Autodesk Inventor part; units mm, degrees
ref_plane "YZ Plane" through (0, 0, 0) normal (1, 0, 0) x (0, 1, 0)
ref_plane "XZ Plane" through (0, 0, 0) normal (0, 1, 0) x (-1, 0, 0)
ref_plane "XY Plane" through (0, 0, 0) normal (0, 0, 1) x (1, 0, 0)
sketch "Sketch1" plane through (0, 0, 0) normal (0, 0, 1) x (1, 0, 0)
  line L0 (0, 0) -> (0, -152.4)
  line L1 (76.2, -152.4) -> (76.2, 0)
  arc A0 (0, -152.4) -> (76.2, -152.4) centre (38.1, -152.4) ccw
  arc A1 (76.2, 0) -> (0, 0) centre (38.1, 0) ccw
  circle A2 centre (38.1, 0) radius 1.5875
  circle A3 centre (38.1, -152.4) radius 1.5875
  dimension "d17" = 3.175
  dimension "d18" = 3.175
extrude "Extrusion1" add sketch "Sketch1" along normal blind 6.35 contours A1 L1 A0 L0 | A2 | A3
extrude "Extrusion4" cut sketch "Sketch1" along normal blind 12.7 contours A2 | A3
sketch "Sketch3" plane through (0, 0, 6.35) normal (0, 0, 1) x (1, 0, 0)
  arc A0 (0, -152.4) -> (76.2, -152.4) centre (38.1, -152.4) ccw
  line L0 (38.1, -190.5) -> (38.1, -187.325)
  arc A1 (3.175, -152.4) -> (38.1, -187.325) centre (38.1, -152.4) ccw
  arc A2 (76.2, 0) -> (0, 0) centre (38.1, 0) ccw
  line L1 (38.1, 38.1) -> (38.1, 34.925)
  arc A3 (38.1, 34.925) -> (3.175, 0) centre (38.1, 0) ccw
  line L2 (3.175, -152.4) -> (3.175, 0)
  line L3 (0, 0) -> (0, -152.4)
  dimension "d21" = 3.175
  dimension "d23" = 3.175
  dimension "d24" = 3.175
extrude "Extrusion5" add sketch "Sketch3" along normal blind 12.7
sketch "Sketch4" plane through (0, 0, 6.35) normal (0, 0, 1) x (1, 0, 0)
  point P0 (0, 0)
properties part number "ChainGuard"
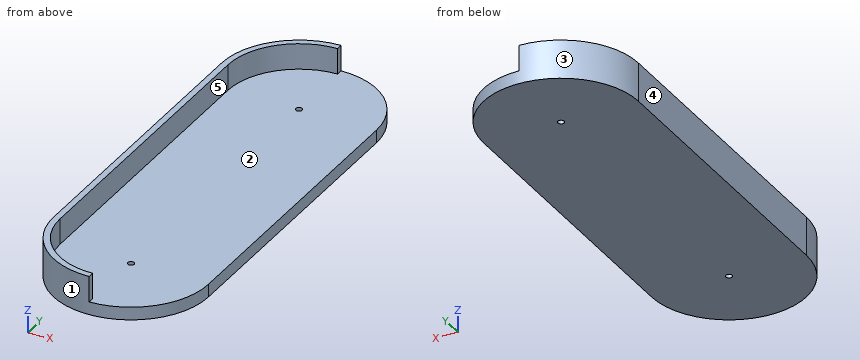
Part model, mm, in its own coordinate system. Face numbers are marked on the shaded views. A direction names the side the tool comes from. Coordinates: 2 decimals unless noted, no trailing zeros. Order: outer loops, then holes, each group sorted by start corner. A loop starts at its lowest first (then second) coordinate and runs counter-clockwise, first axis right, second up.
(1) Slice it at B-B, the plane y = -115. Write the cut outline in (x, z) (3 decimals).
Check sheet entries:
outline: (0, 0) - (76.2, 0) - (76.2, 6.35) - (3.175, 6.35) - (3.175, 19.05) - (0, 19.05) - close
(2) Pull direction Y, two halves, no side cores. Call the marked faces 1, 2 and 3: pulls with the +Y half, pulls with the -Y half, needs draft (parallel to the pull), parting line crosses it, or undercut.
Check sheet entries:
face 1: pulls with the -Y half
face 2: undercut
face 3: pulls with the +Y half
(3) Tool access for the marked faces 4 and 5: list every direction of +Z, -Z, +X, -X, +Y, -Y with a clear straight run to the whole face (end or side of a thin tool).
Check sheet entries:
face 4: +Z, -Z, -X, +Y, -Y
face 5: +Z, +X
(4) Probe L1, parallel to Y at x = 38.1, z = 1.5; L2, parallel to X at y = 0, z = 3.5; L3, parallel to Z at x = 10, y = 13. List the from-to ranges inside material, lowest first.
Check sheet entries:
L1: y = -190.5 to -153.99, -150.81 to -1.59, 1.59 to 38.1
L2: x = 0 to 36.51, 39.69 to 76.2
L3: z = 0 to 6.35
(5) Slice it at A-A, the plane z = 16.5. Write the cut outline in (x, y) (3 decimals).
Check sheet entries:
outline: (0, -152.4) arc R38.1 ccw to (38.1, -190.5) - (38.1, -187.325) arc R34.925 cw to (3.175, -152.4) - (3.175, 0) arc R34.925 cw to (38.1, 34.925) - (38.1, 38.1) arc R38.1 ccw to (0, 0) - close
(6) Pin check, flat tips, straight feed: pin 1 Ø2.5 at (x, y) = (38.1, 0) entering from -Z; pin 2 Ø10 at (x, z) = (63, 5) entering from +Y; pin 3 Ø22 at (x, y) = (39, -117) entering from +Z; pin 4 Ø10 at (x, z) = (13.5, 13.5) entering from +Y. Stop position of each tip, or through.
Check sheet entries:
pin 1: passes through
pin 2: stops at y = 32.49
pin 3: stops at z = 6.35
pin 4: stops at y = 32.67
(7) Slice it at D-D, the plane x = 27. Write the cut outline in (y, z), and give its area (3 significant figures).
Check sheet entries:
outline: (-188.85, 0) - (36.45, 0) - (36.45, 19.05) - (33.11, 19.05) - (33.11, 6.35) - (-185.51, 6.35) - (-185.51, 19.05) - (-188.85, 19.05) - close
area: 1,520 mm2
(8) Slice it at C-C, the plane z = 3.25. Write the cut outline in (x, y) (1 decimal).
Check sheet entries:
outline: (0, -152.4) arc R38.1 ccw to (76.2, -152.4) - (76.2, 0) arc R38.1 ccw to (0, 0) - close; hole circle Ø3.2 at (38.1, -152.4); hole circle Ø3.2 at (38.1, 0)
